Source: CAD feature listing. Evaluate the final solid. Frame: model axes, mm. Give positions to 0.01 mm unless a question says otherwise; leave off trailing zeros. Order: outer loops, then holes, each group sorted by start corner. A loop starts at its lowest first (then second) coordinate and runs counter-clockwise, first axis right, second up. Notation, with made-up numbers: M 77,-7 L 96,-7 A6 ccw 96,-1 Z; hole C 33,-1 d7. An arc over 180 degrees is marked long. Use CSV: the item, a comma, the result in double quotes. Start each with the question number.
Item 1: Section query B-B on z = -37. Return loops of the section in (x, y).
Item 2: Ray query, probe 1 along X at (y, z) = (-3.05, 15); probe 2 along X at (y, z) = (-2.2, 14.5); probe 3 along X at (y, z) = (-2.2, -2). Return the intervals inside material, ascending. Write a range as from..to.
Item 3: Section query A-A on y = -2.4. Count the separate pieces of the cut face and the enclosed holes in it, and give its area (3 significant figures).
Item 4: First-contact query: pin 1 (1.3 mm diameter, centred on y = -3, z = 12.5, fed in from +X); pin 2 (1.5 mm diameter, centred on y = -2, z = -40.5, fed in from -X). Flat tips, straight axial feed; report the tip coordinate or a pass-through.
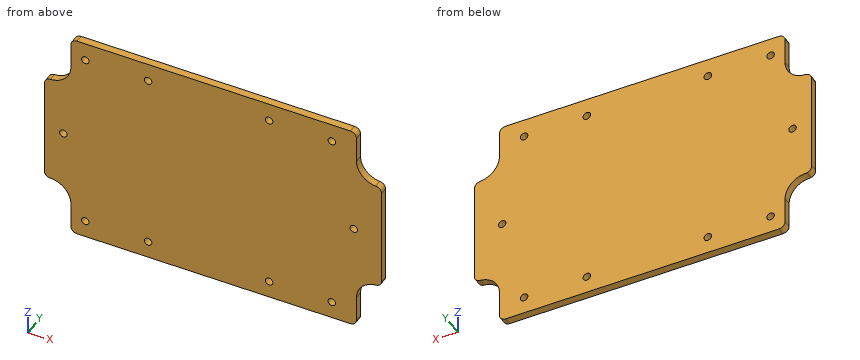
from build123d import *

# Parameters (mm, degrees)
BOSS_EXTRUDE2_DEPTH = 2.54


with BuildPart() as part:
    # Sketch1 → Boss-Extrude2 (new body)
    with BuildSketch(Plane(origin=(0, -3.804704038, 0), x_dir=(1, 0, 0), z_dir=(0, 1, 0))):
        with BuildLine():
            Line((57.814610393, -1.399255471), (57.814610393, 31.463731379))
            add(Edge.make_bspline(
                [(57.814610393, 31.463731379), (57.81461039, 31.720749656), (57.713354059, 32.24087993), (57.283601426, 32.898996274), (56.638589176, 33.350770599), (56.123774909, 33.468351967), (55.867443389, 33.476897959)],
                knots=[0, 0, 0, 0, 0.001152389, 0.002304779, 0.003457168, 0.004609557, 0.004609557, 0.004609557, 0.004609557], degree=3))
            ThreePointArc((55.867443389, 33.476897959), (51.352854042, 35.727909928), (49.531351994, 40.432237951))
            Line((49.531351994, 40.432237951), (49.531351994, 48.932237951))
            ThreePointArc((49.531351994, 48.932237951), (48.94134809, 50.356633378), (47.516952663, 50.946637283))
            Line((47.516952663, 50.946637283), (-42.883047337, 50.946637283))
            ThreePointArc((-42.883047337, 50.946637283), (-44.307442765, 50.356633378), (-44.897446669, 48.932237951))
            Line((-44.897446669, 48.932237951), (-44.897446669, 40.432237951))
            ThreePointArc((-44.897446669, 40.432237951), (-47.052603702, 35.385909486), (-52.188281684, 33.453309044))
            add(Edge.make_bspline(
                [(-52.188281684, 33.453309044), (-52.43565379, 33.383556369), (-52.908782875, 33.144941164), (-53.425568037, 32.552710177), (-53.685335706, 31.809298042), (-53.65878771, 31.281894674), (-53.597446669, 31.032864237)],
                knots=[0, 0, 0, 0, 0.001152389, 0.002304779, 0.003457168, 0.004609557, 0.004609557, 0.004609557, 0.004609557], degree=3))
            Line((-53.597446669, 31.032864237), (-53.597446669, -1.372873912))
            add(Edge.make_bspline(
                [(-53.597446669, -1.372873912), (-53.597446666, -1.629892189), (-53.496190335, -2.150022463), (-53.066437702, -2.808138807), (-52.421425452, -3.259913132), (-51.906611185, -3.3774945), (-51.650279665, -3.386040492)],
                knots=[0, 0, 0, 0, 0.001152389, 0.002304779, 0.003457168, 0.004609557, 0.004609557, 0.004609557, 0.004609557], degree=3))
            ThreePointArc((-51.650279665, -3.386040492), (-46.861860291, -5.511189457), (-44.897446669, -10.367762049))
            Line((-44.897446669, -10.367762049), (-44.897446669, -18.867762049))
            ThreePointArc((-44.897446669, -18.867762049), (-44.307442765, -20.292157477), (-42.883047337, -20.882161381))
            Line((-42.883047337, -20.882161381), (47.516952663, -20.882161381))
            ThreePointArc((47.516952663, -20.882161381), (48.94134809, -20.292157477), (49.531351994, -18.867762049))
            Line((49.531351994, -18.867762049), (49.531351994, -10.367762049))
            ThreePointArc((49.531351994, -10.367762049), (51.352854045, -5.663434025), (55.867443396, -3.412422057))
            add(Edge.make_bspline(
                [(55.867443396, -3.412422057), (56.12431895, -3.403857932), (56.640786427, -3.285326537), (57.284217505, -2.833883412), (57.714248467, -2.174175738), (57.814610385, -1.655729411), (57.814610393, -1.399255471)],
                knots=[0, 0, 0, 0, 0.001152389, 0.002304779, 0.003457168, 0.004609557, 0.004609557, 0.004609557, 0.004609557], degree=3))
        make_face()
        with BuildLine():
            ThreePointArc((20.629561635, 43.959437934), (21.879561635, 45.209437934), (20.629561635, 46.459437934))
            ThreePointArc((20.629561635, 46.459437934), (19.379561635, 45.209437934), (20.629561635, 43.959437934))
        make_face(mode=Mode.SUBTRACT)
        with BuildLine():
            ThreePointArc((41.379561635, 43.959437934), (42.629561635, 45.209437934), (41.379561635, 46.459437934))
            ThreePointArc((41.379561635, 46.459437934), (40.129561635, 45.209437934), (41.379561635, 43.959437934))
        make_face(mode=Mode.SUBTRACT)
        with BuildLine():
            ThreePointArc((48.629561635, 16.459437934), (47.379561635, 15.209437934), (48.629561635, 13.959437934))
            ThreePointArc((48.629561635, 13.959437934), (49.879561635, 15.209437934), (48.629561635, 16.459437934))
        make_face(mode=Mode.SUBTRACT)
        with BuildLine():
            ThreePointArc((41.379561635, -13.540562066), (40.129561635, -14.790562066), (41.379561635, -16.040562066))
            ThreePointArc((41.379561635, -16.040562066), (42.629561635, -14.790562066), (41.379561635, -13.540562066))
        make_face(mode=Mode.SUBTRACT)
        with BuildLine():
            ThreePointArc((20.629561635, -13.540562066), (19.379561635, -14.790562066), (20.629561635, -16.040562066))
            ThreePointArc((20.629561635, -16.040562066), (21.879561635, -14.790562066), (20.629561635, -13.540562066))
        make_face(mode=Mode.SUBTRACT)
        with BuildLine():
            ThreePointArc((-19.370438365, -13.540562066), (-20.620438365, -14.790562066), (-19.370438365, -16.040562066))
            ThreePointArc((-19.370438365, -16.040562066), (-18.120438365, -14.790562066), (-19.370438365, -13.540562066))
        make_face(mode=Mode.SUBTRACT)
        with BuildLine():
            ThreePointArc((-40.120438365, -16.040562066), (-38.870438365, -14.790562066), (-40.120438365, -13.540562066))
            ThreePointArc((-40.120438365, -13.540562066), (-41.370438365, -14.790562066), (-40.120438365, -16.040562066))
        make_face(mode=Mode.SUBTRACT)
        with BuildLine():
            ThreePointArc((-47.370438365, 13.959437934), (-46.120438365, 15.209437934), (-47.370438365, 16.459437934))
            ThreePointArc((-47.370438365, 16.459437934), (-48.620438365, 15.209437934), (-47.370438365, 13.959437934))
        make_face(mode=Mode.SUBTRACT)
        with BuildLine():
            ThreePointArc((-40.120438365, 43.959437934), (-38.870438365, 45.209437934), (-40.120438365, 46.459437934))
            ThreePointArc((-40.120438365, 46.459437934), (-41.370438365, 45.209437934), (-40.120438365, 43.959437934))
        make_face(mode=Mode.SUBTRACT)
        with BuildLine():
            ThreePointArc((-19.370438365, 43.959437934), (-18.120438365, 45.209437934), (-19.370438365, 46.459437934))
            ThreePointArc((-19.370438365, 46.459437934), (-20.620438365, 45.209437934), (-19.370438365, 43.959437934))
        make_face(mode=Mode.SUBTRACT)
    extrude(amount=BOSS_EXTRUDE2_DEPTH)


solid = part.part
Verdict:
1,outline,"M -45.8,-3.8 L 50.43,-3.8 L 50.43,-1.26 L -45.8,-1.26 Z"
2,probe 1,"-44.9..-41.35, -38.89..-20.6, -18.14..19.4, 21.86..40.15, 42.61..49.53"
2,probe 2,"-44.9..-41.34, -38.9..-20.59, -18.15..19.41, 21.85..40.16, 42.6..49.53"
2,probe 3,"-53.6..57.81"
3,separate pieces,"1"
3,enclosed holes,"10"
3,area,"7,390 mm2"
4,pin 1,"x = 49.53"
4,pin 2,"x = -44.93"
